```python
from build123d import *

# Parameters (mm, degrees)
SKETCH1_W                      = 100
SKETCH1_H                      = 100
SKETCH1_W_2                    = 94
SKETCH1_H_2                    = 94
EXTRUDE_THIN1_DEPTH            = 130
FILLET1_R                      = 0.5
FILLET2_R                      = 3
F_8_0_8_DIAMETER_HOLE2_D       = 8
F_8_0_8_DIAMETER_HOLE3_D       = 8
F_10_0_10_DIAMETER_HOLE1_D     = 10
F_10_0_10_DIAMETER_HOLE2_D     = 10
M8X1_25_TAPPED_HOLE1_D         = 6.8
M8X1_25_TAPPED_HOLE1_DEPTH     = 3
M8X1_25_TAPPED_HOLE2_D         = 6.8
M8X1_25_TAPPED_HOLE2_DEPTH     = 3
F_21_0_21_DIAMETER_HOLE1_D     = 21
F_21_0_21_DIAMETER_HOLE1_DEPTH = 3
F_5_0_5_DIAMETER_HOLE1_D       = 5
F_5_0_5_DIAMETER_HOLE1_DEPTH   = 3
F_8_0_8_DIAMETER_HOLE4_D       = 8
F_8_0_8_DIAMETER_HOLE4_DEPTH   = 3
CUT_EXTRUDE1_REACH             = 173.464
SKETCH31_R                     = 2
SKETCH31_R_2                   = 3.5
F_8_0_8_DIAMETER_HOLE5_D       = 8
F_8_0_8_DIAMETER_HOLE5_DEPTH   = 3


with BuildPart() as part:
    # Sketch1 → Extrude-Thin1 (new body)
    with BuildSketch(Plane.XY):
        Rectangle(SKETCH1_W, SKETCH1_H)
        Rectangle(SKETCH1_W_2, SKETCH1_H_2, mode=Mode.SUBTRACT)
    extrude(amount=EXTRUDE_THIN1_DEPTH)

    # Fillet1
    fillet1_edges = [part.edges().sort_by_distance(p)[0] for p in [
        (47, -47, 65),
        (47, 47, 65),
        (-47, 47, 65),
        (-47, -47, 65),
    ]]
    fillet(fillet1_edges, radius=FILLET1_R)

    # Fillet2
    fillet2_edges = [part.edges().sort_by_distance(p)[0] for p in [
        (50, -50, 65),
        (-50, -50, 65),
        (-50, 50, 65),
        (50, 50, 65),
    ]]
    fillet(fillet2_edges, radius=FILLET2_R)

    # Ø8.0 (8) Diameter Hole2 (through all)
    with Locations(Plane(origin=(0, 50, 0), x_dir=(1, 0, 0), z_dir=(0, 1, 0))):
        with Locations((28, -32), (28, -90)):
            Hole(F_8_0_8_DIAMETER_HOLE2_D / 2)

    # Ø8.0 (8) Diameter Hole3 (through all)
    with Locations(Plane(origin=(50, 0, 0), x_dir=(0, 0, -1), z_dir=(1, 0, 0))):
        with Locations((-14, 31), (-110, 31)):
            Hole(F_8_0_8_DIAMETER_HOLE3_D / 2)

    # Ø10.0 (10) Diameter Hole1 (through all)
    with Locations(Plane(origin=(0, 50, 0), x_dir=(1, 0, 0), z_dir=(0, 1, 0))):
        with Locations((-34, -56)):
            Hole(F_10_0_10_DIAMETER_HOLE1_D / 2)

    # Ø10.0 (10) Diameter Hole2 (through all)
    with Locations(Plane(origin=(50, 0, 0), x_dir=(0, 0, -1), z_dir=(1, 0, 0))):
        with Locations((-44, -31)):
            Hole(F_10_0_10_DIAMETER_HOLE2_D / 2)

    # M8x1.25 Tapped Hole1
    with Locations(Plane.ZY.offset(50)):
        with Locations((56, -15), (56, 35)):
            Hole(M8X1_25_TAPPED_HOLE1_D / 2, depth=M8X1_25_TAPPED_HOLE1_DEPTH)

    # M8x1.25 Tapped Hole2
    with Locations(Plane(origin=(0, -50, 0), x_dir=(-1, 0, 0), z_dir=(0, -1, 0))):
        with Locations((20, -44), (-35, -44)):
            Hole(M8X1_25_TAPPED_HOLE2_D / 2, depth=M8X1_25_TAPPED_HOLE2_DEPTH)

    # Ø21.0 (21) Diameter Hole1
    with Locations(Plane(origin=(50, 0, 0), x_dir=(0, 0, -1), z_dir=(1, 0, 0))):
        with Locations((-70, 0)):
            Hole(F_21_0_21_DIAMETER_HOLE1_D / 2, depth=F_21_0_21_DIAMETER_HOLE1_DEPTH)

    # Ø5.0 (5) Diameter Hole1
    with Locations(Plane(origin=(50, 0, 0), x_dir=(0, 0, -1), z_dir=(1, 0, 0))):
        with Locations((-41.157258279, -16.652364697), (-53.347635303, 28.842741721), (-98.842741721, 16.652364697), (-86.652364697, -28.842741721)):
            Hole(F_5_0_5_DIAMETER_HOLE1_D / 2, depth=F_5_0_5_DIAMETER_HOLE1_DEPTH)

    # Ø8.0 (8) Diameter Hole4
    with Locations(Plane(origin=(0, 50, 0), x_dir=(1, 0, 0), z_dir=(0, 1, 0))):
        with Locations((-3, -25)):
            Hole(F_8_0_8_DIAMETER_HOLE4_D / 2, depth=F_8_0_8_DIAMETER_HOLE4_DEPTH)

    # Sketch31 → Cut-Extrude1 (cut, up to next)
    with BuildSketch(Plane(origin=(50, 0, 0), x_dir=(0, 0, -1), z_dir=(1, 0, 0)), mode=Mode.PRIVATE) as cut_extrude1_sk1:
        with Locations(Location((-5, 4, 0), (0, 0, 90))):
            Circle(SKETCH31_R)
    cut_extrude1_tool1 = extrude(cut_extrude1_sk1.sketch, amount=-CUT_EXTRUDE1_REACH, mode=Mode.PRIVATE) & part.part
    # Sketch31 → Cut-Extrude1 (cut, up to next)
    with BuildSketch(Plane(origin=(50, 0, 0), x_dir=(0, 0, -1), z_dir=(1, 0, 0)), mode=Mode.PRIVATE) as cut_extrude1_sk2:
        with Locations(Location((-5, 13, 0), (0, 0, 90))):
            Circle(SKETCH31_R)
    cut_extrude1_tool2 = extrude(cut_extrude1_sk2.sketch, amount=-CUT_EXTRUDE1_REACH, mode=Mode.PRIVATE) & part.part
    # Sketch31 → Cut-Extrude1 (cut, up to next)
    with BuildSketch(Plane(origin=(50, 0, 0), x_dir=(0, 0, -1), z_dir=(1, 0, 0)), mode=Mode.PRIVATE) as cut_extrude1_sk3:
        with Locations(Location((-125, 13, 0), (0, 0, 90))):
            Circle(SKETCH31_R)
    cut_extrude1_tool3 = extrude(cut_extrude1_sk3.sketch, amount=-CUT_EXTRUDE1_REACH, mode=Mode.PRIVATE) & part.part
    # Sketch31 → Cut-Extrude1 (cut, up to next)
    with BuildSketch(Plane(origin=(50, 0, 0), x_dir=(0, 0, -1), z_dir=(1, 0, 0)), mode=Mode.PRIVATE) as cut_extrude1_sk4:
        with Locations(Location((-125, 4, 0), (0, 0, 90))):
            Circle(SKETCH31_R)
    cut_extrude1_tool4 = extrude(cut_extrude1_sk4.sketch, amount=-CUT_EXTRUDE1_REACH, mode=Mode.PRIVATE) & part.part
    # Sketch31 → Cut-Extrude1 (cut, up to next)
    with BuildSketch(Plane(origin=(50, 0, 0), x_dir=(0, 0, -1), z_dir=(1, 0, 0)), mode=Mode.PRIVATE) as cut_extrude1_sk5:
        with Locations(Location((-23, 8.5, 0), (0, 0, 90))):
            Circle(SKETCH31_R_2)
    cut_extrude1_tool5 = extrude(cut_extrude1_sk5.sketch, amount=-CUT_EXTRUDE1_REACH, mode=Mode.PRIVATE) & part.part
    # Sketch31 → Cut-Extrude1 (cut, up to next)
    with BuildSketch(Plane(origin=(50, 0, 0), x_dir=(0, 0, -1), z_dir=(1, 0, 0)), mode=Mode.PRIVATE) as cut_extrude1_sk6:
        with Locations(Location((-107, 8.5, 0), (0, 0, 90))):
            Circle(SKETCH31_R_2)
    cut_extrude1_tool6 = extrude(cut_extrude1_sk6.sketch, amount=-CUT_EXTRUDE1_REACH, mode=Mode.PRIVATE) & part.part
    add(cut_extrude1_tool1.solids().sort_by_distance((50, 4, 5))[0], mode=Mode.SUBTRACT)
    add(cut_extrude1_tool2.solids().sort_by_distance((50, 13, 5))[0], mode=Mode.SUBTRACT)
    add(cut_extrude1_tool3.solids().sort_by_distance((50, 13, 125))[0], mode=Mode.SUBTRACT)
    add(cut_extrude1_tool4.solids().sort_by_distance((50, 4, 125))[0], mode=Mode.SUBTRACT)
    add(cut_extrude1_tool5.solids().sort_by_distance((50, 8.5, 23))[0], mode=Mode.SUBTRACT)
    add(cut_extrude1_tool6.solids().sort_by_distance((50, 8.5, 107))[0], mode=Mode.SUBTRACT)

    # Ø8.0 (8) Diameter Hole5
    with Locations(Plane(origin=(0, 50, 0), x_dir=(1, 0, 0), z_dir=(0, 1, 0))):
        with Locations((-33, -25)):
            Hole(F_8_0_8_DIAMETER_HOLE5_D / 2, depth=F_8_0_8_DIAMETER_HOLE5_DEPTH)


solid = part.part
```
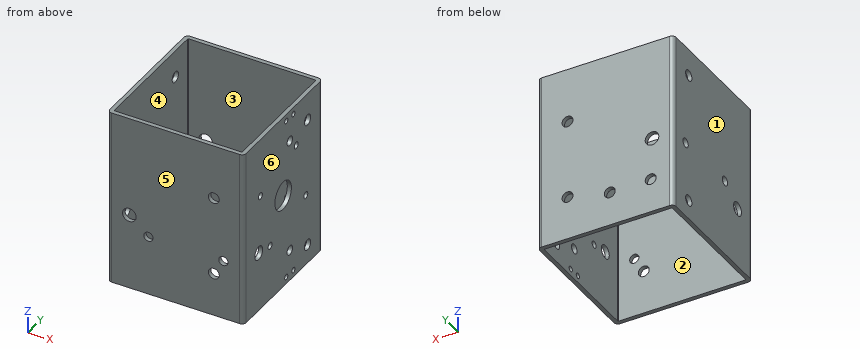
Model file for the job. Use its own axes, mm. Face numbers are marked on the shaded views. A direction names the side the tool comes from. Give positions to 0.01 mm unless a question says otherwise; leave off trailing zeros. Write each loop counter-clockwise with the first axis right and the second up, starting at its lowest first coordinate (ties: lowest second). Pieces come first, ordered by that corner, then holes. Notation, with made-up numbers: (-8.5, -5) -> (-0.5, -5) arc R18 cw to (-0.5, 17) -> close; hole circle Ø7 at (88, 14.25). An arc over 180 degrees is marked (long way). Use CSV: the item, a comma, the result in double quotes. Start each with the question number.
1) Pin check, flat tips, straight feed: P1, Ø6.5, axis at y = 16.65, z = 98.84, coming from the +X side; P2, Ø5, axis at x = 28, z = 32, coming from the -Y side; P3, Ø7, axis at x = -3, z = 25, coming from the +Y side; P4, Ø6.5, axis at y = 8.5, z = 107, coming from the +X side. Stop position of each tip, or through.
2) Drill centre lines: L1, parallel to Z at x = 28, y = -49.25; L2, parallel to Y at x = -28, z = 85. Where is each one in solid material? Low to high.
3) Cut at D-D on z = 70. List the corners of the cut face in (x, y), plus the area to 3 significant figures.
4) Cut at B-B on z = 32. List the corners of the cut face in (x, y).
5) Cut at A-A on x = -26. List the corners of the cut face in (y, z).
6) Two-plate mould, pull along X, no slides. Class the marked faces 3, 4, 5 and 6: released by +X, released by -X, zero draft, split by the parting line, or undercut.
7) Cut at C-C on x = 35. List the corners of the cut face in (y, z).
8) Tool access for the marked faces 1 and 2: list every direction of +Z, -Z, +X, -X, +Y, -Y with a clear straight run to the whole face (end or side of a thin tool).
Final values:
1,P1,"stops at x = 50"
1,P2,"passes through"
1,P3,"stops at y = -47"
1,P4,"stops at x = -47"
2,L1,"z = 0 to 28, 36 to 86, 94 to 130"
2,L2,"y = -50 to -47, 47 to 50"
3,outline,"(-50, -47) arc R3 ccw to (-47, -50) -> (47, -50) arc R3 ccw to (50, -47) -> (50, -10.5) -> (47, -10.5) -> (47, -46.5) arc R0.5 cw to (46.5, -47) -> (-46.5, -47) arc R0.5 cw to (-47, -46.5) -> (-47, 46.5) arc R0.5 cw to (-46.5, 47) -> (46.5, 47) arc R0.5 cw to (47, 46.5) -> (47, 10.5) -> (50, 10.5) -> (50, 47) arc R3 ccw to (47, 50) -> (-47, 50) arc R3 ccw to (-50, 47) -> close"
3,area,"1,090 mm2"
4,outline,"(-50, -47) arc R3 ccw to (-47, -50) -> (24, -50) -> (24, -47) -> (-46.5, -47) arc R0.5 cw to (-47, -46.5) -> (-47, 46.5) arc R0.5 cw to (-46.5, 47) -> (24, 47) -> (24, 50) -> (-47, 50) arc R3 ccw to (-50, 47) -> close; (32, -50) -> (47, -50) arc R3 ccw to (50, -47) -> (50, 47) arc R3 ccw to (47, 50) -> (32, 50) -> (32, 47) -> (46.5, 47) arc R0.5 cw to (47, 46.5) -> (47, -46.5) arc R0.5 cw to (46.5, -47) -> (32, -47) -> close"
5,outline,"(-50, 0) -> (-47, 0) -> (-47, 130) -> (-50, 130) -> close; (47, 0) -> (50, 0) -> (50, 130) -> (47, 130) -> close"
6,face 3,"undercut"
6,face 4,"undercut"
6,face 5,"zero draft"
6,face 6,"released by +X"
7,outline,"(-50, 0) -> (-47, 0) -> (-47, 40.6) -> (-50, 40.6) -> close; (-50, 47.4) -> (-47, 47.4) -> (-47, 130) -> (-50, 130) -> close; (47, 0) -> (50, 0) -> (50, 130) -> (47, 130) -> close"
8,face 1,"+Z, -Z, -X, +Y, -Y"
8,face 2,"+Z, -Z"
